Geometry check sheet. Reference: the model listing, model coordinates, mm. Coordinates: 2 decimals unless noted, no trailing zeros. Write each loop counter-clockwise with the first axis right and the second up, starting at its lowest first coordinate (ties: lowest second). Pieces come first, ordered by that corner, then holes. Notation, with made-up numbers: (47.25, 63) -> (59.25, 63) arc R26 ccw to (59.25, 102) -> close; hole circle Ø2 at (15, 37.25). An arc over 180 degrees is marked (long way). One line per question, with ' | ' between items.
```python
from build123d import *

# Parameters (mm, degrees)
BOSS_EXTRUDE1_DEPTH = 5
SKETCH2_W           = 30
SKETCH2_H           = 70
CUT_EXTRUDE1_DEPTH  = 5
CUT_EXTRUDE2_DEPTH  = 5
SKETCH5_R           = 2.5
CUT_EXTRUDE3_DEPTH  = 5
SKETCH6_R           = 2.5
CUT_EXTRUDE4_DEPTH  = 5
CUT_EXTRUDE5_DEPTH  = 5
SKETCH8_R           = 1.5
CUT_EXTRUDE6_DEPTH  = 5


with BuildPart() as part:
    # Sketch1 → Boss-Extrude1 (new body)
    with BuildSketch(Plane.XY):
        with BuildLine():
            Line((-90, -100), (90, -100))
            ThreePointArc((90, -100), (97.071067812, -97.071067812), (100, -90))
            Line((100, -90), (100, 70))
            ThreePointArc((100, 70), (91.213203436, 91.213203436), (70, 100))
            Line((70, 100), (-70, 100))
            ThreePointArc((-70, 100), (-91.213203436, 91.213203436), (-100, 70))
            Line((-100, 70), (-100, -90))
            ThreePointArc((-100, -90), (-97.071067812, -97.071067812), (-90, -100))
        make_face()
    extrude(amount=BOSS_EXTRUDE1_DEPTH)

    # Sketch2 → Cut-Extrude1 (cut)
    with BuildSketch(Plane.XY.offset(5)):
        with Locations((85, -55)):
            Rectangle(SKETCH2_W, SKETCH2_H)
        with Locations((-85, -55)):
            Rectangle(SKETCH2_W, SKETCH2_H)
    extrude(amount=-CUT_EXTRUDE1_DEPTH, mode=Mode.SUBTRACT)

    # Sketch3 → Cut-Extrude2 (cut)
    with BuildSketch(Plane.XY.offset(5)):
        with BuildLine():
            Line((85, -20), (100, -20))
            Line((100, -20), (100, 70))
            add(Edge.make_bspline(
                [(100, 70), (41.562750789, 76.769648156), (85, -20)],
                knots=[0, 0, 0, 1, 1, 1], degree=2))
        make_face()
        with BuildLine():
            Line((-85, -20), (-100, -20))
            Line((-100, -20), (-100, 70))
            add(Edge.make_bspline(
                [(-100, 70), (-41.562750789, 76.769648156), (-85, -20)],
                knots=[0, 0, 0, 1, 1, 1], degree=2))
        make_face()
    extrude(amount=-CUT_EXTRUDE2_DEPTH, mode=Mode.SUBTRACT)

    # Sketch5 → Cut-Extrude3 (cut)
    with BuildSketch(Plane.XY.offset(5)):
        with Locations((50, -80)):
            Circle(SKETCH5_R)
        with Locations((-50, -80)):
            Circle(SKETCH5_R)
        with Locations(Location((50, -20, 0), (0, 0, 180))):
            Circle(SKETCH5_R)
        with Locations(Location((-50, -20, 0), (0, 0, 180))):
            Circle(SKETCH5_R)
    extrude(amount=-CUT_EXTRUDE3_DEPTH, mode=Mode.SUBTRACT)

    # Sketch6 → Cut-Extrude4 (cut)
    with BuildSketch(Plane.XY.offset(5)):
        with Locations((0, -90)):
            Circle(SKETCH6_R)
    extrude(amount=-CUT_EXTRUDE4_DEPTH, mode=Mode.SUBTRACT)

    # Sketch7 → Cut-Extrude5 (cut)
    with BuildSketch(Plane.XY.offset(5)):
        Polygon((-70.182426877, 60), (70.182426877, 60), (160.134720298, 60), (160.134720298, -117.07554651), (-141.914902021, -117.07554651), (-141.914902021, 60), align=None)
    extrude(amount=-CUT_EXTRUDE5_DEPTH, mode=Mode.SUBTRACT)

    # Sketch8 → Cut-Extrude6 (cut)
    with BuildSketch(Plane.XY.offset(5)):
        with Locations((-80, 80)):
            Circle(SKETCH8_R)
        with Locations((80, 80)):
            Circle(SKETCH8_R)
    extrude(amount=-CUT_EXTRUDE6_DEPTH, mode=Mode.SUBTRACT)


solid = part.part
```
(1) Depth check by flat-ended pin: P1, Ø3, axis at y = 86, z = 2.5, coming from the +X side. Enter the tip coordinate at first touch or a pass-through.
Answers below:
P1: stops at x = 96.26
(2) Cross-section at A-A (y = 94). Record the cut outline in (x, z), plus the area to 3 significant figures.
Answers below:
outline: (-88, 0) -> (88, 0) -> (88, 5) -> (-88, 5) -> close | area: 880 mm²
(3) Material ranges on line 1 (X direction, y = 80, z = 2.55); line 2 (Y direction, x = 80, z = 3.6); line 3 (Y direction, x = 82, z = 0.9), recorded low to high.
Answers below:
line 1: x = -98.28 to -81.5, -78.5 to 78.5, 81.5 to 98.28 | line 2: y = 68.3 to 78.5, 81.5 to 98.28 | line 3: y = 69 to 97.5
